Autodesk Inventor part; units mm, degrees
ref_plane "Work Plane1" through (1.525, 0, 0) normal (0, 0, 1) x (1, 0, 0)
ref_plane "YZ Plane" through (0, 0, 0) normal (1, 0, 0) x (0, 1, 0)
ref_plane "XZ Plane" through (0, 0, 0) normal (0, 1, 0) x (-1, 0, 0)
sketch "Sketch1" plane through (0, 0, 0) normal (0, 0, 1) x (1, 0, 0)
  line L0 (0, 2.5) -> (0, 1.25)
  line L1 (1.3, 1.25) -> (6, 1.25)
  line L2 (6, 1.25) -> (6, 0)
  line L3 (6, 0) -> (-0.0011, 0)
  line L4 (-1.2013, 0) -> (7.2002, 0)
  line L5 (-0.0011, 0) -> (-0.0011, 2.5)
  line L6 (-0.0011, 2.5) -> (0, 2.5)
  line L7 (1.3, 1.25) -> (1.0238, 1.25)
  line L8 (1.0238, 1.25) -> (0, 1.25)
  line L9 (0, -0.5) -> (0, 3)
  dimension "d0" = 6
  dimension "d1" = 4.7
  dimension "d2" = 2.5
  dimension "d9" = 0.0011
  dimension "d10" = 5
  dimension "d13" = 0.2762
  dimension "d14" = 2.5
revolve "Body" add sketch "Sketch1" angle 360 about axis through (6, 0, 0) along (-1, 0, 0)
sketch "Sketch2" plane through (-0.0011, 0, 0) normal (-1, 0, 0) x (0, 0, 1)
  line L0 (0, 2.8868) -> (2.5, 1.4434)
  line L1 (2.5, 1.4434) -> (2.5, -1.4434)
  line L2 (2.5, -1.4434) -> (0, -2.8868)
  line L3 (0, -2.8868) -> (-2.5, -1.4434)
  line L4 (-2.5, -1.4434) -> (-2.5, 1.4434)
  line L5 (-2.5, 1.4434) -> (0, 2.8868)
  point P0 (0, 0)
  point P1 (0, 0)
  dimension "d11" = 5
extrude "Head" add sketch "Sketch2" along normal blind 10
sketch "Sketch4" plane through (0, 0, 0) normal (0, 0, 1) x (1, 0, 0)
  line L0 (-10.0011, 2.5) -> (-10.0011, 2.8868)
  line L1 (-10.0011, 2.8868) -> (-9.7778, 2.8868)
  line L2 (-9.7778, 2.8868) -> (-10.0011, 2.5)
  line L3 (-2.0399, 0) -> (0.3387, 0)
  line L4 (-0.0011, 2.8868) -> (-10.0011, 2.8868)
  line L5 (-10.0011, 1.4434) -> (-10.0011, 2.8868)
  dimension "d5" = 30
  dimension "d19" = 5
revolve "Chamfer1" cut sketch "Sketch4" angle 360 about axis through (-10, 0, 0) along (1, 0, 0)
thread "Thread"
chamfer "Chamfer2" distance 0.2761 distance2 0.2762 1 edges at (6, -1.25, 0) measured on face at (6, -0.3871, 0.3429)
ref_plane "Work Plane1" through (1.525, 0, 0) normal (0, 0, 1) x (1, 0, 0)
sketch "Sketch7" plane through (-10.0011, 0, 0) normal (-1, 0, 0) x (0, 0, 1)
  circle A0 centre (0, 0) radius 1.45
  point P0 (0, 0)
  dimension "d59" = 2.9
extrude "Extrusion5" cut sketch "Sketch7" against normal blind 5
equation "\"d11\" = SW"
equation "\"d15\" = GEL"
equation "\"d6\" = -0.5 * SPD + 0.5 * GD"
equation "\"d0\" = NLG"
equation "\"d1\" = GEL"
equation "\"d2\" = GD"
equation "\"d10\" = SD2"
equation "\"d14\" = BDM"
equation "\"d5\" = ANG1"
equation "\"d19\" = SW0"
equation "\"NLG\" = 6"
equation "\"GD\" = NND"
equation "\"BDM\" = NND"
equation "\"KOH\" = 1.7"
equation "\"GEL\" = 4.7"
equation "\"SW\" = 5"
equation "\"SW0\" = SW"
equation "\"SPD\" = NND - 1.2269 * PTC"
equation "\"SD2\" = SW"
equation "\"SD\" = 0.001"
equation "\"ANG1\" = 30deg"
equation "\"GAL\" = 0.61345 * PTC"
equation "\"GUL\" = 0.61345 * PTC"
equation "\"RR\" = 0.001"
equation "\"WFT\" = SD"
equation "\"GD1\" = THREADDIA - 1.2269 * PTC"
equation "\"THREADDIA\" = 2.5"
equation "\"SDH\" = SW"
equation "\"TOA\" = 30deg"
equation "\"FAWI\" = 45deg"
equation "\"PTC\" = 0.45"
equation "\"NND\" = 2.5"
equation "\"E0\" = 1.155 * SW"
properties part number "AS 1110 - M2.5 x 6" material "Steel, Mild"
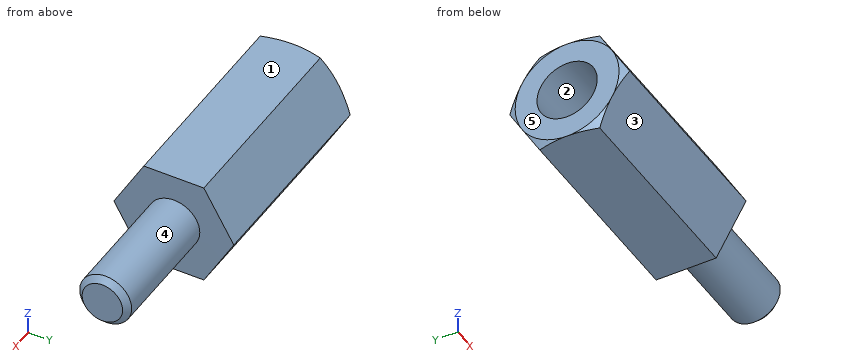
Verification items for the finished model (mm, model axes). Face numbers are marked on the shaded views. A direction names the side the tool comes from. Coordinates: 2 decimals unless noted, no trailing zeros. Write each loop counter-clockwise with the first axis right and the second up, starting at its lowest first coordinate (ties: lowest second). Pieces come first, ordered by that corner, then holes. Notation, with made-up numbers: M -0.5,73 L 36.5,73 A17 cw 36.5,106 Z; hole C 75,-5 d1. An arc over 180 degrees is marked long. Answer as a JSON object with one key per item and string values. Group by question number.
(1) Cross-section at C-C, the plane x = 0.5. Record the cut outline in (y, z).
(2) Cross-section at A-A, the plane x = -8.25. Record the cut outline in (y, z), and give its area (3 significant figures).
(3) Material ranges on line 1 (Z direction, x = -9, y = 0.1); line 2 (X direction, y = -0.6, z = 0.6); line 3 (X direction, y = 1.7, z = 0.9), recorded low to high.
(4) Gauge pin test, flat end, axial feed: pin 1 (2.5 mm diameter, centred on y = 0, z = 0, fed in from -X). Record the tip position at first contact, or that the pin passes through.
(5) Release check for a two-part mould opening along Z. For the marked faces 1, 2 and 3 record: +Z half, -Z half, draft (parallel to the pull), parting line (faces both ways), or undercut.
(6) Tool access check on the marked faces 4 and 5. Record the directions out of +Z, -Z, +X, -X, +Y, -Y that give a thin tool (end or side, any length) a straight path to the whole face; none if there is none.
(7) Cross-section at B-B, the plane x = -4.5. Record the cut outline in (y, z).
Reply:
{
 "1": {"outline": "C 0,0 d2.5"},
 "2": {"outline": "M -2.89,0 L -1.44,-2.5 L 1.44,-2.5 L 2.89,0 L 1.44,2.5 L -1.44,2.5 Z; hole C 0,0 d2.9", "area": "15.0 mm²"},
 "3": {"line 1": "-2.5 to -1.45, 1.45 to 2.5", "line 2": "-5 to 6", "line 3": "-10 to 0"},
 "4": {"pin 1": "x = -5"},
 "5": {"face 1": "+Z half", "face 2": "undercut", "face 3": "-Z half"},
 "6": {"face 4": "+X", "face 5": "+Z, -Z, -X, +Y, -Y"},
 "7": {"outline": "M -2.89,0 L -1.44,-2.5 L 1.44,-2.5 L 2.89,0 L 1.44,2.5 L -1.44,2.5 Z"}
}
